from build123d import *

# Parameters (mm, degrees)
SKETCH1_W           = 31.75
SKETCH1_H           = 63.5
SKETCH1_W_2         = 25.4
SKETCH1_H_2         = 57.15
BOSS_EXTRUDE1_DEPTH = 838.2
CUT_EXTRUDE1_REACH  = 843.015
SKETCH2_R           = 9.525
SKETCH2_R_2         = 2.54


with BuildPart() as part:
    # Sketch1 → Boss-Extrude1 (new body)
    with BuildSketch(Plane.XY):
        with Locations((3.710272719, -29.23968021)):
            Rectangle(SKETCH1_W, SKETCH1_H)
        with Locations((3.710272719, -29.23968021)):
            Rectangle(SKETCH1_W_2, SKETCH1_H_2, mode=Mode.SUBTRACT)
    extrude(amount=BOSS_EXTRUDE1_DEPTH)

    # Cut-Extrude1: up to this face of the body (flat: up to its plane)
    cut_extrude1_end = Plane(part.part.faces().sort_by_distance((-12.164727281, -29.23968021, 419.1))[0])
    # Sketch2 → Cut-Extrude1 (cut, up to the picked face)
    with BuildSketch(Plane(origin=(19.585272719, 0, 0), x_dir=(0, 0, -1), z_dir=(1, 0, 0)), mode=Mode.PRIVATE) as cut_extrude1_sk1:
        with Locations(Location((-752.475, -29.23968021, 0), (0, 0, 90))):
            Circle(SKETCH2_R)
    cut_extrude1_tool1 = split(extrude(cut_extrude1_sk1.sketch, amount=-CUT_EXTRUDE1_REACH, mode=Mode.PRIVATE), bisect_by=cut_extrude1_end, keep=Keep.BOTH, mode=Mode.PRIVATE)
    # Sketch2 → Cut-Extrude1 (cut, up to the picked face)
    with BuildSketch(Plane(origin=(19.585272719, 0, 0), x_dir=(0, 0, -1), z_dir=(1, 0, 0)), mode=Mode.PRIVATE) as cut_extrude1_sk2:
        with Locations(Location((-752.475, -48.28968021, 0), (0, 0, 90))):
            Circle(SKETCH2_R_2)
    cut_extrude1_tool2 = split(extrude(cut_extrude1_sk2.sketch, amount=-CUT_EXTRUDE1_REACH, mode=Mode.PRIVATE), bisect_by=cut_extrude1_end, keep=Keep.BOTH, mode=Mode.PRIVATE)
    # Sketch2 → Cut-Extrude1 (cut, up to the picked face)
    with BuildSketch(Plane(origin=(19.585272719, 0, 0), x_dir=(0, 0, -1), z_dir=(1, 0, 0)), mode=Mode.PRIVATE) as cut_extrude1_sk3:
        with Locations(Location((-752.475, -10.18968021, 0), (0, 0, 90))):
            Circle(SKETCH2_R_2)
    cut_extrude1_tool3 = split(extrude(cut_extrude1_sk3.sketch, amount=-CUT_EXTRUDE1_REACH, mode=Mode.PRIVATE), bisect_by=cut_extrude1_end, keep=Keep.BOTH, mode=Mode.PRIVATE)
    # Sketch2 → Cut-Extrude1 (cut, up to the picked face)
    with BuildSketch(Plane(origin=(19.585272719, 0, 0), x_dir=(0, 0, -1), z_dir=(1, 0, 0)), mode=Mode.PRIVATE) as cut_extrude1_sk4:
        with Locations(Location((-85.725, -48.28968021, 0), (0, 0, 270))):
            Circle(SKETCH2_R_2)
    cut_extrude1_tool4 = split(extrude(cut_extrude1_sk4.sketch, amount=-CUT_EXTRUDE1_REACH, mode=Mode.PRIVATE), bisect_by=cut_extrude1_end, keep=Keep.BOTH, mode=Mode.PRIVATE)
    # Sketch2 → Cut-Extrude1 (cut, up to the picked face)
    with BuildSketch(Plane(origin=(19.585272719, 0, 0), x_dir=(0, 0, -1), z_dir=(1, 0, 0)), mode=Mode.PRIVATE) as cut_extrude1_sk5:
        with Locations(Location((-85.725, -29.23968021, 0), (0, 0, 270))):
            Circle(SKETCH2_R)
    cut_extrude1_tool5 = split(extrude(cut_extrude1_sk5.sketch, amount=-CUT_EXTRUDE1_REACH, mode=Mode.PRIVATE), bisect_by=cut_extrude1_end, keep=Keep.BOTH, mode=Mode.PRIVATE)
    # Sketch2 → Cut-Extrude1 (cut, up to the picked face)
    with BuildSketch(Plane(origin=(19.585272719, 0, 0), x_dir=(0, 0, -1), z_dir=(1, 0, 0)), mode=Mode.PRIVATE) as cut_extrude1_sk6:
        with Locations(Location((-85.725, -10.18968021, 0), (0, 0, 270))):
            Circle(SKETCH2_R_2)
    cut_extrude1_tool6 = split(extrude(cut_extrude1_sk6.sketch, amount=-CUT_EXTRUDE1_REACH, mode=Mode.PRIVATE), bisect_by=cut_extrude1_end, keep=Keep.BOTH, mode=Mode.PRIVATE)
    add(cut_extrude1_tool1.solids().sort_by(Axis((19.585273, -29.23968, 752.475), (-1, 0, 0)))[0], mode=Mode.SUBTRACT)
    add(cut_extrude1_tool2.solids().sort_by(Axis((19.585273, -48.28968, 752.475), (-1, 0, 0)))[0], mode=Mode.SUBTRACT)
    add(cut_extrude1_tool3.solids().sort_by(Axis((19.585273, -10.18968, 752.475), (-1, 0, 0)))[0], mode=Mode.SUBTRACT)
    add(cut_extrude1_tool4.solids().sort_by(Axis((19.585273, -48.28968, 85.725), (-1, 0, 0)))[0], mode=Mode.SUBTRACT)
    add(cut_extrude1_tool5.solids().sort_by(Axis((19.585273, -29.23968, 85.725), (-1, 0, 0)))[0], mode=Mode.SUBTRACT)
    add(cut_extrude1_tool6.solids().sort_by(Axis((19.585273, -10.18968, 85.725), (-1, 0, 0)))[0], mode=Mode.SUBTRACT)


solid = part.part
Work out the finished part from the listing and answer in its coordinate system (mm). A direction names the side the tool comes from. Round coordinates to 2 decimals unless told otherwise and drop trailing zeros. Write each loop counter-clockwise with the first axis right and the second up, starting at its lowest first coordinate (ties: lowest second). Pieces come first, ordered by that corner, then holes.
1) A cutting plane is placed at C-C (y = -27.5). Give the vertices of the cut face in (x, z), plus the area to 3 significant figures.
2) A cutting plane is placed at A-A (x = 3). Give the vertices of the cut face in (y, z), plus the area to 3 significant figures.
3) Given pin 1 Ø4.5 at (y, z) = (-10.19, 85.72) entering from +X; pin 2 Ø25 at (y, z) = (-29.24, 85.72) entering from -X, each flat-ended and moving along its own axis, determine where each tip first touches the part or whether it passes through.
4) The mould has two halves that part along X. Classify faces 1 (the flat face through (16.41, -30, 413)), 2 (the flat face through (-12.165, -30, 413)), 3 (the flat face through (3, -60.99, 413)): pulls with the +X half, pulls with the -X half, needs draft (parallel to the pull), parting line crosses it, or undercut.
5) A cutting plane is placed at B-B (z = 637.5). Give the vertices of the cut face in (x, y).
6) A tool of negligible diameter and unlimited length cuts with its end or side. For faces 4 (the flat face through (-9.3, -26.7, 0)), 5 (the flat face through (4, -0.665, 413)), from which of +Z, -Z, +X, -X, +Y, -Y can it reach the whole face along a straight path? Write none if from no direction.
7) Straight lines are drawn through the part: line 1 (Z direction, x = -10.5, y = -48); line 2 (X direction, y = -28.5, z = 637); line 3 (Y direction, x = -4, z = 320). For each, find the intervals that lie inside material, in ascending order.
Completed:
1. outline: (-12.16, 0) - (-8.99, 0) - (-8.99, 76.36) - (-12.16, 76.36) - close; (-12.16, 95.09) - (-8.99, 95.09) - (-8.99, 743.11) - (-12.16, 743.11) - close; (-12.16, 761.84) - (-8.99, 761.84) - (-8.99, 838.2) - (-12.16, 838.2) - close; (16.41, 0) - (19.59, 0) - (19.59, 76.36) - (16.41, 76.36) - close; (16.41, 95.09) - (19.59, 95.09) - (19.59, 743.11) - (16.41, 743.11) - close; (16.41, 761.84) - (19.59, 761.84) - (19.59, 838.2) - (16.41, 838.2) - close
1. area: 5,080 mm2
2. outline: (-60.99, 0) - (-57.81, 0) - (-57.81, 838.2) - (-60.99, 838.2) - close; (-0.66, 0) - (2.51, 0) - (2.51, 838.2) - (-0.66, 838.2) - close
2. area: 5,320 mm2
3. pin 1: passes through
3. pin 2: stops at x = -12.16
4. face 1: undercut
4. face 2: pulls with the -X half
4. face 3: needs draft
5. outline: (-12.16, -60.99) - (19.59, -60.99) - (19.59, 2.51) - (-12.16, 2.51) - close; hole (-8.99, -57.81) - (16.41, -57.81) - (16.41, -0.66) - (-8.99, -0.66) - close
6. face 4: -Z, +X, -X, +Y, -Y
6. face 5: +Z, -Z
7. line 1: z = 0 to 83.2, 88.25 to 749.95, 755 to 838.2
7. line 2: x = -12.16 to -8.99, 16.41 to 19.59
7. line 3: y = -60.99 to -57.81, -0.66 to 2.51
